Part model, mm, in its own coordinate system. A direction names the side the tool comes from. Give positions to 0.01 mm unless a question says otherwise; leave off trailing zeros. Order: outer loops, then holes, each group sorted by start corner. A loop starts at its lowest first (then second) coordinate and runs counter-clockwise, first axis right, second up.
1. Slice it at D-D on y = 34.5. List the corners of the cut face in (x, z).
2. Which spindle directions (+Z, -Z, +X, -X, +Y, -Y) get a long thin tool onto all of the face, cutting with end or side? Do faces 1 (the flat face through (149, -10, 1)), 2 (the flat face through (22, 29, -50)). Say none if no direction does.
3. Slice it at A-A on y = 0. List the corners of the cut face in (x, z).
4. Slice it at B-B on x = 162.5. List the corners of the cut face in (y, z).
5. Slice it at C-C on z = 16.5. List the corners of the cut face in (x, y), and give its area (3 significant figures).
6. Probe line 1 (X direction, y = 4, z = -32); line 2 (Y direction, x = 0, z = 14); line 3 (Y direction, x = 118, z = -12.5). List the from-to ranges inside material, lowest first.
7. Drop flat-ended pins along their axis: pin 1 Ø6 at (y, z) = (8, -13) entering from -X; pin 2 Ø8 at (x, z) = (67, 35.5) entering from +Y; pin 3 Ø8 at (x, z) = (151, 25) entering from +Y. Give the stop position or say it passes through.
8. Mould opens along X. For faces 3 (the cylindrical face through (-46.916, 98.906, -0.7)), 4 (the cylindrical face through (-61.32, 114.55, 0.7)), 5 (the cylindrical face through (-14.985, 0.66, -0.7)), 6 (the flat face through (178.762, 15, 1)) say: +X half, -X half, draft (parallel to the pull), parting line (faces both ways), or undercut.
from build123d import *

# Parameters (mm, degrees)
SKETCH3_R           = 15
SKETCH3_R_2         = 10
BOSS_EXTRUDE1_DEPTH = 50


with BuildPart() as part:
    # Sketch3 → Boss-Extrude1 (new, symmetric)
    with BuildSketch(Plane.XY):
        with BuildLine():
            ThreePointArc((-28.016593122, -10.72709233), (-17.002753161, -24.716520486), (0, -30))
            Line((0, -30), (178.761781376, -30))
            Line((178.761781376, -30), (178.761781376, -10))
            Line((178.761781376, -10), (118.761781376, -10))
            ThreePointArc((118.761781376, -10), (108.761781376, 0), (118.761781376, 10))
            Line((118.761781376, 10), (178.761781376, 10))
            Line((178.761781376, 10), (178.761781376, 20))
            ThreePointArc((178.761781376, 20), (68.667725633, 45.525627999), (-24.170625815, 109.971724042))
            ThreePointArc((-24.170625815, 109.971724042), (-61.804778357, 114.246632888), (-73.630323726, 78.263848671))
            Line((-73.630323726, 78.263848671), (-70.680690942, 72.509208706))
            Line((-70.680690942, 72.509208706), (-28.016593122, -10.72709233))
        make_face()
        Circle(SKETCH3_R, mode=Mode.SUBTRACT)
        with Locations((-45.613730605, 88.990941002)):
            Circle(SKETCH3_R_2, mode=Mode.SUBTRACT)
    extrude(amount=BOSS_EXTRUDE1_DEPTH, both=True)


solid = part.part
Data:
1. outline: (-51.2, -50) - (97.44, -50) - (97.44, 50) - (-51.2, 50) - close
2. face 1: +Z, -Z, +X
2. face 2: -Z, +X, -X, +Y, -Y
3. outline: (-33.51, -50) - (-15, -50) - (-15, 50) - (-33.51, 50) - close; (15, -50) - (108.76, -50) - (108.76, 50) - (15, 50) - close
4. outline: (-30, -50) - (-10, -50) - (-10, 50) - (-30, 50) - close; (10, -50) - (21.07, -50) - (21.07, 50) - (10, 50) - close
5. outline: (-73.63, 78.26) - (-28.02, -10.73) arc R30 ccw to (0, -30) - (178.76, -30) - (178.76, -10) - (118.76, -10) arc R10 cw to (118.76, 10) - (178.76, 10) - (178.76, 20) arc R300 cw to (-24.17, 109.97) arc R30 ccw to start; hole circle Ø20 at (-45.61, 88.99); hole circle Ø30 at (0, 0)
5. area: 17,900 mm2
6. line 1: x = -35.57 to -14.46, 14.46 to 109.6
6. line 2: y = -30 to -15, 15 to 87.83
6. line 3: y = -30 to -9.97, 9.97 to 28.61
7. pin 1: stops at x = -39.15
7. pin 2: stops at y = 48.11
7. pin 3: stops at y = 22.92
8. face 3: undercut
8. face 4: parting line
8. face 5: undercut
8. face 6: +X half
